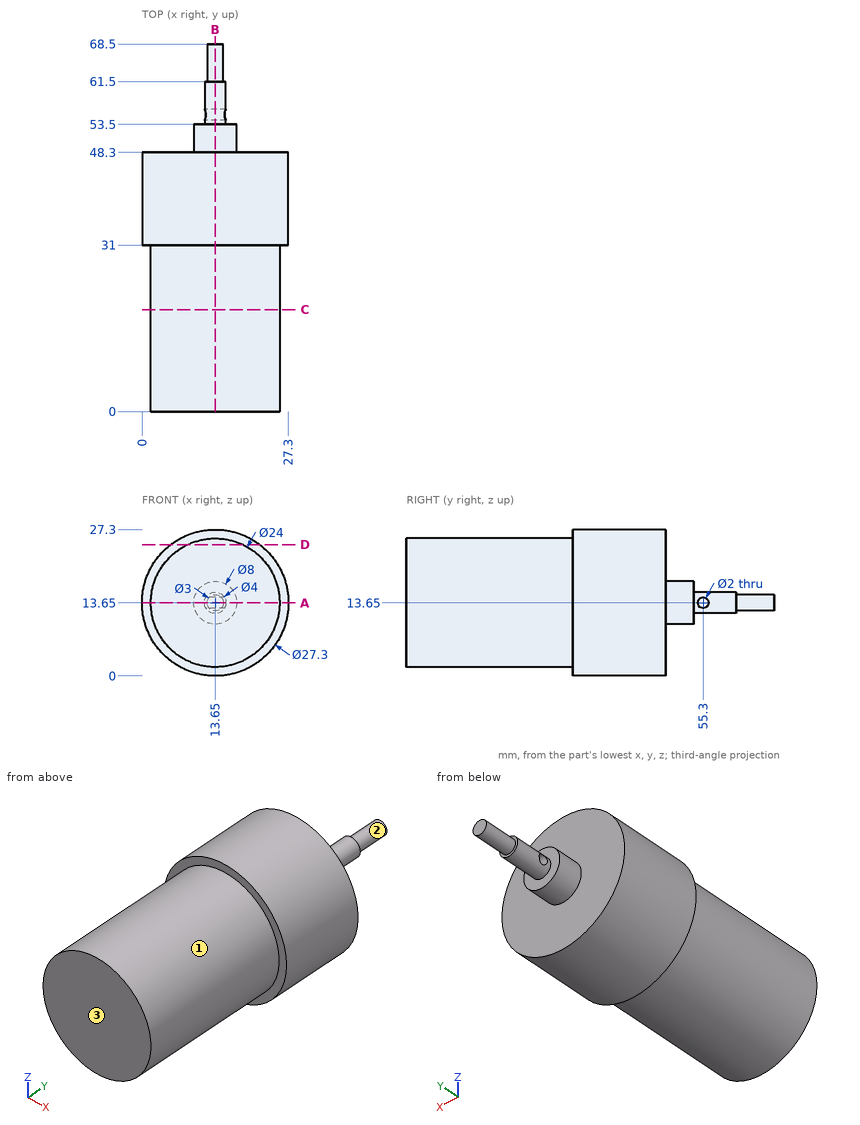
The drawing under review shows one solid part. Ordinate dimensions are in mm from its lowest x, y, z. A direction names the side the tool comes from. Give positions to 0.01 mm unless a question says otherwise; leave off trailing zeros. Order: outer loops, then holes, each group sorted by start corner. A loop starts at its lowest first (then second) coordinate and runs counter-clockwise, first axis right, second up. Notation, with made-up numbers: M 17,47.25 L 68,47.25 A13 ccw 68,51.25 Z; hole C 28,-17.75 d6. An arc over 180 degrees is marked long. One line per question, with ' | ' between items. Start each with the question number.
Q1. For L1, parallel to Z at x = 13.7, y = 55.3; L2, parallel to Y at x = 16.75, z = 5.75; L3, parallel to Y at x = 12.85, z = 13.65, list the stretches that pass through material, from the lowest coordinate up. Write a range as [from, to].
Q2. Machinability: for the marked faces 1, 2 and 3, which of the approach directions +Z, -Z, +X, -X, +Y, -Y give a long, thin tool a straight path to every point of the face, cutting with its end or side? Answer none if there is none.
Q3. We need section B-B (x = 13.65). Write out the cut boundary in (y, z).
Q4. We need section A-A (z = 13.65). Write out the cut boundary in (x, y), plus the area to 3 significant figures.
Q5. We need section C-C (y = 19). Write out the cut boundary in (x, z).
Q6. We need section D-D (z = 24.5). Write out the cut boundary in (x, y), plus the area to 3 significant figures.
Q7. For pin 1 Ø12 at (x, y) = (6, 10.5) entering from +Z; pin 2 Ø2 at (x, y) = (6, 21) entering from -Z; pin 3 Ø1.8 at (y, z) = (55.3, 13.65) entering from -X; pin 4 Ø12 at (x, y) = (22, 36.5) entering from -Z, all flat-tipped, find the tip position at first contact; note any pin that passes through.
Returned:
1) L1: [11.65, 12.65], [14.65, 15.65] | L2: [0, 48.3] | L3: [0, 54.3], [56.3, 68.5]
2) face 1: -Y | face 2: +Y | face 3: +Z, -Z, +X, -X, -Y
3) outline: M 0,1.65 L 31,1.65 L 31,0 L 48.3,0 L 48.3,9.65 L 53.5,9.65 L 53.5,11.65 L 61.5,11.65 L 61.5,12.15 L 68.5,12.15 L 68.5,15.15 L 61.5,15.15 L 61.5,15.65 L 53.5,15.65 L 53.5,17.65 L 48.3,17.65 L 48.3,27.3 L 31,27.3 L 31,25.65 L 0,25.65 Z; hole C 55.3,13.65 d2
4) outline: M 0,31 L 1.65,31 L 1.65,0 L 25.65,0 L 25.65,31 L 27.3,31 L 27.3,48.3 L 17.65,48.3 L 17.65,53.5 L 15.65,53.5 L 15.65,54.3 L 11.65,54.3 L 11.65,53.5 L 9.65,53.5 L 9.65,48.3 L 0,48.3 Z; M 11.65,56.3 L 15.65,56.3 L 15.65,61.5 L 15.15,61.5 L 15.15,68.5 L 12.15,68.5 L 12.15,61.5 L 11.65,61.5 Z | area: 1,300 mm2
5) outline: C 13.65,13.65 d24
6) outline: M 5.37,31 L 8.52,31 L 8.52,0 L 18.78,0 L 18.78,31 L 21.93,31 L 21.93,48.3 L 5.37,48.3 Z | area: 604 mm2
7) pin 1: z = 25.54 | pin 2: z = 3.66 | pin 3: through | pin 4: z = 0.2
